from build123d import *

# Parameters (mm, degrees)
SKETCH3_R           = 29.5
BOSS_EXTRUDE4_DEPTH = 7
CUT_EXTRUDE1_DEPTH  = 3.6
SKETCH5_R           = 7.5
CUT_EXTRUDE2_DEPTH  = 11.8
CUT_EXTRUDE3_DEPTH  = 15.8
SKETCH7_R           = 1.75
CUT_EXTRUDE4_DEPTH  = 20
SKETCH8_R           = 3.75
CUT_EXTRUDE5_DEPTH  = 2.4


with BuildPart() as part:
    # Sketch3 → Boss-Extrude4 (new body)
    with BuildSketch(Plane(origin=(0, 0, 0), x_dir=(1, 0, 0), z_dir=(0, 1, 0))):
        Circle(SKETCH3_R)
    extrude(amount=BOSS_EXTRUDE4_DEPTH)

    # Sketch4 → Cut-Extrude1 (cut)
    with BuildSketch(Plane(origin=(0, 7, 0), x_dir=(1, 0, 0), z_dir=(0, 1, 0))):
        with BuildLine():
            Line((-3.4, 24.6), (-3.4, 15))
            Line((-3.4, 15), (-7.194348327, 2.119281046))
            ThreePointArc((-7.194348327, 2.119281046), (0, -7.5), (7.194348327, 2.119281046))
            Line((7.194348327, 2.119281046), (3.4, 15))
            Line((3.4, 15), (3.4, 24.6))
            ThreePointArc((3.4, 24.6), (0, 28), (-3.4, 24.6))
        make_face()
    extrude(amount=-CUT_EXTRUDE1_DEPTH, mode=Mode.SUBTRACT)

    # Sketch5 → Cut-Extrude2 (cut)
    with BuildSketch(Plane(origin=(0, 7, 0), x_dir=(1, 0, 0), z_dir=(0, 1, 0))):
        Circle(SKETCH5_R)
        with BuildLine():
            Line((3, 24.5), (3, 20.5))
            ThreePointArc((3, 20.5), (0, 17.5), (-3, 20.5))
            Line((-3, 20.5), (-3, 24.5))
            ThreePointArc((-3, 24.5), (0, 27.5), (3, 24.5))
        make_face()
    extrude(amount=-CUT_EXTRUDE2_DEPTH, mode=Mode.SUBTRACT)

    # Sketch6 → Cut-Extrude3 (cut)
    with BuildSketch(Plane(origin=(0, 7, 0), x_dir=(1, 0, 0), z_dir=(0, 1, 0))):
        with BuildLine():
            Line((20.392959569, 10.493464633), (32.610697072, 22.711202135))
            Line((32.610697072, 22.711202135), (22.711202135, 32.610697072))
            Line((22.711202135, 32.610697072), (10.493464633, 20.392959569))
            ThreePointArc((10.493464633, 20.392959569), (10.493464633, 10.493464633), (20.392959569, 10.493464633))
        make_face()
        with BuildLine():
            Line((10.493464633, -20.392959569), (22.711202135, -32.610697072))
            Line((22.711202135, -32.610697072), (32.610697072, -22.711202135))
            Line((32.610697072, -22.711202135), (20.392959569, -10.493464633))
            ThreePointArc((20.392959569, -10.493464633), (10.493464633, -10.493464633), (10.493464633, -20.392959569))
        make_face()
        with BuildLine():
            Line((-20.392959569, -10.493464633), (-32.610697072, -22.711202135))
            Line((-32.610697072, -22.711202135), (-22.711202135, -32.610697072))
            Line((-22.711202135, -32.610697072), (-10.493464633, -20.392959569))
            ThreePointArc((-10.493464633, -20.392959569), (-10.493464633, -10.493464633), (-20.392959569, -10.493464633))
        make_face()
        with BuildLine():
            Line((-10.493464633, 20.392959569), (-22.711202135, 32.610697072))
            Line((-22.711202135, 32.610697072), (-32.610697072, 22.711202135))
            Line((-32.610697072, 22.711202135), (-20.392959569, 10.493464633))
            ThreePointArc((-20.392959569, 10.493464633), (-10.493464633, 10.493464633), (-10.493464633, 20.392959569))
        make_face()
    extrude(amount=-CUT_EXTRUDE3_DEPTH, mode=Mode.SUBTRACT)

    # Sketch7 → Cut-Extrude4 (cut)
    with BuildSketch(Plane(origin=(116.330739936, 17, -202.28312586), x_dir=(0.707106781, 0, 0.707106781), z_dir=(0, 1, 0))):
        with Locations((74.91965057, -211.151889461)):
            Circle(SKETCH7_R)
        with Locations((74.91965057, -239.436160708)):
            Circle(SKETCH7_R)
        with Locations((46.635379323, -239.436160708)):
            Circle(SKETCH7_R)
    extrude(amount=-CUT_EXTRUDE4_DEPTH, mode=Mode.SUBTRACT)

    # Sketch8 → Cut-Extrude5 (cut)
    with BuildSketch(Plane.XZ):
        with Locations((0, 20)):
            Circle(SKETCH8_R)
        with Locations((20, 0)):
            Circle(SKETCH8_R)
        with Locations((-20, 0)):
            Circle(SKETCH8_R)
    extrude(amount=-CUT_EXTRUDE5_DEPTH, mode=Mode.SUBTRACT)


solid = part.part
The listing builds one solid part. Answer for the finished solid, in the listing's coordinates (mm). A direction names the side the tool comes from. Give positions to 0.01 mm unless a question says otherwise; leave off trailing zeros. Write each loop counter-clockwise with the first axis right and the second up, starting at its lowest first coordinate (ties: lowest second). Pieces come first, ordered by that corner, then holes.
1) Section B-B (y = 1.5) is taken. Write down the section's boundary in (x, z).
2) Find the intervals of material crossed by L1, parallel to Z at x = 0, y = 0.5; L2, parallel to X at y = 4, z = 0; L3, parallel to Z at x = -15, y = 6.5, in increasing order.
3) Section C-C (z = 19) is taken. Write down the section's boundary in (x, y).
4) Given P1, Ø3, axis at x = -20, z = 0, coming from the -Y side; P2, Ø3, axis at y = 4.5, z = -20.5, coming from the -X side; P3, Ø4, axis at x = 20.5, z = -0.5, coming from the -Y side; P4, Ø2, axis at x = 13, z = 9.5, coming from the +Y side, each flat-ended and moving along its own axis, determine where each tip first touches the part or whether it passes through.
5) For a pull along X with two mould halves and no side action, classify faces 1 (the face through (6, 0, 6)), 2 (the face through (3, 2, -23)), 3 (the face through (29.5, 3.5, 0.2)) as pulls with the +X half, pulls with the -X half, needs draft (parallel to the pull), parting line crosses it, or undercut.
6) Section A-A (x = 0) is taken. Write down the section's boundary in (y, z), and give its area (3 significant figures).
7) A tool of negligible diameter and unlimited length cuts with its end or side. For faces 4 (the face through (-0.81, 1.18, 16.34)), 5 (the face through (12.9, 3.5, -22.8)), 6 (the face through (-12.9, 3.5, -22.8)), 7 (the face through (22.8, 3.5, -12.9)), 8 (the face through (5.324, 5.225, -8.469)), from which of +Z, -Z, +X, -X, +Y, -Y can it reach the whole face along a straight path? Write none if from no direction.
8) Section D-D (x = -6) is taken. Write down the section's boundary in (y, z), and give its area (3 significant figures).
Response:
1. outline: (-25.21, -15.31) - (-20.39, -10.49) arc R7 cw to (-10.49, -20.39) - (-15.31, -25.21) arc R29.5 ccw to (15.31, -25.21) - (10.49, -20.39) arc R7 cw to (20.39, -10.49) - (25.21, -15.31) arc R29.5 ccw to (25.21, 15.31) - (20.39, 10.49) arc R7 cw to (10.49, 20.39) - (15.31, 25.21) arc R29.5 ccw to (-15.31, 25.21) - (-10.49, 20.39) arc R7 cw to (-20.39, 10.49) - (-25.21, 15.31) arc R29.5 ccw to start; hole circle Ø7.5 at (-20, 0); hole circle Ø15 at (0, 0); hole circle Ø7.5 at (0, 20); hole (-3, -24.5) arc R3 ccw to (3, -24.5) - (3, -20.5) arc R3 ccw to (-3, -20.5) - close; hole circle Ø7.5 at (20, 0)
2. L1: z = -29.5 to -27.5, -17.5 to -7.5, 7.5 to 16.25, 23.75 to 29.5
2. L2: x = -29.5 to -21.75, -18.25 to -7.5, 7.5 to 18.25, 21.75 to 29.5
2. L3: z = -25.4 to -24.9, -8.46 to 8.46, 24.9 to 25.4
3. outline: (-9.41, 0) - (-3.61, 0) - (-3.61, 2.4) - (-1.44, 2.4) - (-1.44, 7) - (-9.41, 7) - close; (1.44, 2.4) - (3.61, 2.4) - (3.61, 0) - (9.41, 0) - (9.41, 7) - (1.44, 7) - close
4. P1: passes through
4. P2: stops at x = -12.1
4. P3: stops at y = 2.4
4. P4: stops at y = 7
5. face 1: needs draft
5. face 2: undercut
5. face 3: pulls with the +X half
6. outline: (0, -29.5) - (7, -29.5) - (7, -28) - (3.4, -28) - (3.4, -27.5) - (0, -27.5) - close; (0, -17.5) - (3.4, -17.5) - (3.4, -7.5) - (0, -7.5) - close; (0, 7.5) - (7, 7.5) - (7, 18.25) - (2.4, 18.25) - (2.4, 16.25) - (0, 16.25) - close; (0, 23.75) - (2.4, 23.75) - (2.4, 21.75) - (7, 21.75) - (7, 29.5) - (0, 29.5) - close
6. area: 166 mm2
7. face 4: -Y
7. face 5: +X, +Y, -Y
7. face 6: -X, +Y, -Y
7. face 7: -Z, +Y, -Y
7. face 8: +Y
8. outline: (0, -28.88) - (7, -28.88) - (7, -6.17) - (3.4, -6.17) - (3.4, -4.5) - (0, -4.5) - close; (0, 4.5) - (7, 4.5) - (7, 28.88) - (0, 28.88) - close
8. area: 335 mm2
